```python
from build123d import *

# Parameters (mm, degrees)
SKETCH1_W           = 27
SKETCH1_H           = 27
SKETCH1_R           = 1.75
BOSS_EXTRUDE1_DEPTH = 4.5
SKETCH1_3_W         = 10
SKETCH1_3_H         = 8
BOSS_EXTRUDE2_DEPTH = 15.75
FILLET1_R           = 10
SKETCH2_R           = 2.55
CUT_EXTRUDE1_DEPTH  = 28.795008545
FILLET2_RADIUS      = 4
FILLET2_LENGTH      = 10
FILLET3_R           = 3
CUT_EXTRUDE2_DEPTH  = 3
FILLET6_R           = 3


with BuildPart() as part:
    # Sketch1 → Boss-Extrude1 (new body)
    with BuildSketch(Plane.XY):
        Rectangle(SKETCH1_W, SKETCH1_H)
        with Locations((-9.5, 8)):
            Circle(SKETCH1_R, mode=Mode.SUBTRACT)
        with Locations((9.5, 8)):
            Circle(SKETCH1_R, mode=Mode.SUBTRACT)
    extrude(amount=BOSS_EXTRUDE1_DEPTH)

    # Sketch1<3> → Boss-Extrude2 (add)
    with BuildSketch(Plane.XY):
        Rectangle(SKETCH1_3_W, SKETCH1_3_H)
    extrude(amount=BOSS_EXTRUDE2_DEPTH)

    # Fillet1
    fillet1_edges = [part.edges().sort_by_distance(p)[0] for p in [
        (-13.5, -13.5, 2.25),
        (13.5, -13.5, 2.25),
    ]]
    fillet(fillet1_edges, radius=FILLET1_R)

    # Sketch2 → Cut-Extrude1 (cut, through all)
    with BuildSketch(Plane.ZY.offset(5)):
        with Locations((11.75, 0)):
            Circle(SKETCH2_R)
    extrude(amount=-CUT_EXTRUDE1_DEPTH, mode=Mode.SUBTRACT)

    # Fillet2: full round fillet: the end face becomes a half cylinder, R = half its width
    fillet2_face = Plane((0, 0, 15.75), x_dir=(-1, 0, 0), z_dir=(0, 0, 1))  # on the end face: x along it, z out of the body
    fillet2_slab = fillet2_face.offset(-FILLET2_RADIUS / 2) * Box(FILLET2_LENGTH, 2 * FILLET2_RADIUS, FILLET2_RADIUS, mode=Mode.PRIVATE)  # the body's end, R deep
    fillet2_round = Plane((0, 0, 11.75), x_dir=(0, 0, 1), z_dir=(-1, 0, 0)) * Cylinder(FILLET2_RADIUS, FILLET2_LENGTH, mode=Mode.PRIVATE)  # its axis R under the face
    add(fillet2_slab - fillet2_round, mode=Mode.SUBTRACT)

    # Fillet3
    fillet3_edges = [part.edges().sort_by_distance(p)[0] for p in [
        (0, -4, 4.5),
        (0, 4, 4.5),
    ]]
    fillet(fillet3_edges, radius=FILLET3_R)

    # Sketch3 → Cut-Extrude2 (cut)
    with BuildSketch(Plane.XY.offset(4.5)):
        Polygon((-9.5, 12.5033321), (-13.4, 10.25166605), (-13.4, 5.74833395), (-9.5, 3.4966679), (-5.6, 5.74833395), (-5.6, 10.25166605), align=None)
        Polygon((5.6, 10.25166605), (9.5, 12.5033321), (13.4, 10.25166605), (13.4, 5.74833395), (9.5, 3.4966679), (5.6, 5.74833395), align=None)
    extrude(amount=-CUT_EXTRUDE2_DEPTH, mode=Mode.SUBTRACT)

    # Fillet6
    fillet6_edges = [part.edges().sort_by_distance(p)[0] for p in [
        (-13.5, 13.5, 2.25),
        (13.5, 13.5, 2.25),
    ]]
    fillet(fillet6_edges, radius=FILLET6_R)


solid = part.part
```
For this review, take the finished solid that the model builds, in its own axes (mm). A direction names the side the tool comes from. Coordinates: 2 decimals unless noted, no trailing zeros. Order: outer loops, then holes, each group sorted by start corner. A loop starts at its lowest first (then second) coordinate and runs counter-clockwise, first axis right, second up. Notation, with made-up numbers: (58.5, 0.5) - (67.5, 0.5) arc R23 cw to (67.5, 15.5) - close; hole circle Ø3 at (48.25, 27). An arc over 180 degrees is marked (long way). Answer as a JSON object with one key per item and string values. Group by question number.
1. For faces 1 (the flat face through (11.423, 11.393, 3.021)), 2 (the cylindrical face through (12.6, 12.64, 2.28)), list the 3-axis set-ups (+Z, -Z, +X, -X, +Y, -Y) from which the entire face can be reached by the end or side of a thin tool; tool diameter is ignored.
2. The part is to be moulded in two halves that separate along Y. For faces 3 (the flat face through (-11.48, 4.64, 3.02)), 4 (the cylindrical face through (-10.65, -10.49, 2.28)), 5 (the flat face through (-11.423, 11.393, 3.021)), 6 (the flat face through (-5, 0, 9)), say which applies: pulls with the +Y half, pulls with the -Y half, needs draft (parallel to the pull), parting line crosses it, or undercut.
3. Clearance check with flat-ended pins moving along their axes: P1, Ø6, axis at x = -11.5, y = 9.5, coming from the +Z side; P2, Ø3.5, axis at x = -0.5, z = 10, coming from the -Y side; P3, Ø5.5, axis at y = 0, z = 11, coming from the +X side; P4, Ø3, axis at x = -9.5, y = 8, coming from the +Z side. State where each tip first meets the part, or that it passes through.
4. We need section C-C on x = 8.5. State the section outline as (y, z) points.
5. We need section D-D on y = 9. State the section outline as (x, z) points.
6. We need section A-A on z = 10.5. State the section outline as (x, y) points, then the cut area to 3 significant figures.
7. For probe 1 along X at (y, z) = (8, 0.9); probe 2 along Y at (x, z) = (2.75, 11.75); probe 3 along Z at (x, y) = (6.25, 9), list the stretches that pass through material, from the lowest coordinate up.
8. We need section B-B on y = 0. State the section outline as (x, z) points, then the cut area to 3 significant figures.
Final values:
{
 "1": {"face 1": "+Z", "face 2": "+Z, -Z, +X, +Y"},
 "2": {"face 3": "undercut", "face 4": "pulls with the -Y half", "face 5": "undercut", "face 6": "needs draft"},
 "3": {"P1": "z = 4.5", "P2": "y = -4", "P3": "x = 5", "P4": "through"},
 "4": {"outline": "(-12.16, 0) - (6.56, 0) - (6.56, 1.5) - (4.07, 1.5) - (4.07, 4.5) - (-12.16, 4.5) - close; (9.44, 0) - (13.5, 0) - (13.5, 4.5) - (11.93, 4.5) - (11.93, 1.5) - (9.44, 1.5) - close"},
 "5": {"outline": "(-13.5, 0) - (-10.94, 0) - (-10.94, 1.5) - (-13.4, 1.5) - (-13.4, 4.5) - (-13.5, 4.5) - close; (-8.06, 0) - (8.06, 0) - (8.06, 1.5) - (5.6, 1.5) - (5.6, 4.5) - (-5.6, 4.5) - (-5.6, 1.5) - (-8.06, 1.5) - close; (10.94, 0) - (13.5, 0) - (13.5, 4.5) - (13.4, 4.5) - (13.4, 1.5) - (10.94, 1.5) - close"},
 "6": {"outline": "(-5, -4) - (5, -4) - (5, -2.22) - (-5, -2.22) - close; (-5, 2.22) - (5, 2.22) - (5, 4) - (-5, 4) - close", "area": "35.5 mm²"},
 "7": {"probe 1": "-13.5 to -11.25, -7.75 to 7.75, 11.25 to 13.5", "probe 2": "-4 to -2.55, 2.55 to 4", "probe 3": "0 to 1.5"},
 "8": {"outline": "(-13.5, 0) - (13.5, 0) - (13.5, 4.5) - (5, 4.5) - (5, 9.2) - (-5, 9.2) - (-5, 4.5) - (-13.5, 4.5) - close; (-5, 14.3) - (5, 14.3) - (5, 15.75) - (-5, 15.75) - close", "area": "183 mm²"}
}
